Can you work these out from the model? Positions are in its coordinate system, mm. A direction names the side the tool comes from. Give positions to 0.01 mm unless a question says otherwise; leave off trailing zeros. Write each loop counter-clockwise with the first axis right and the second up, starting at its lowest first coordinate (ties: lowest second). Pieces come first, ordered by that corner, then holes.
from build123d import *

# Parameters (mm, degrees)
F0_W     = 50
F0_H     = 186
F1_DEPTH = 2
F2_W     = 50
F2_H     = 26
F2_R     = 5
F2_H_2   = 4
F3_DEPTH = 4
F4_W     = 50
F4_H     = 60
F5_DEPTH = 5


with BuildPart() as f1:
    # F0 (on Front) → F1 (new body, symmetric)
    with BuildSketch(Plane.XZ):
        with Locations((0.1773070544, -2)):
            Rectangle(F0_W, F0_H)
    extrude(amount=F1_DEPTH, both=True)

    # F2 (on face) → F3 (join)
    with BuildSketch(Plane.XY.offset(91)):
        with Locations((0.1773070544, 15)):
            Rectangle(F2_W, F2_H)
        with Locations((0.1773070544, 13)):
            Circle(F2_R, mode=Mode.SUBTRACT)
        with Locations((0.1773070544, 0)):
            Rectangle(F2_W, F2_H_2)
    extrude(amount=F3_DEPTH)

    # F4 (on face) → F5 (join)
    with BuildSketch(Plane.XZ.offset(2)):
        with Locations((0.1773070544, -65)):
            Rectangle(F4_W, F4_H)
    extrude(amount=F5_DEPTH)


solid = f1.part
(1) If I drill on L1, parallel to Z at x = -7.5, y = 24; L2, parallel to Y at x = 4.5, z = -31.5; L3, parallel to Y at x = -8, z = -75, over which ranges is the centre line in solid material (lowest first)?
Returned:
L1: z = 91 to 95
L2: y = -2 to 2
L3: y = -7 to 2
(2) Will these pins go through, and if not, where does the flat tip stop? P1, Ø6, axis at x = -5, z = -5.5, coming from the +Y side; P2, Ø10, axis at x = 11.5, z = 1, coming from the -Y side.
Returned:
P1: stops at y = 2
P2: stops at y = -2
(3) Imagine slicing it at B-B, the plane x = 1. Write out the boundary of the cut face in (y, z), plus the area to 3 significant figures.
Returned:
outline: (-7, -95) - (2, -95) - (2, 91) - (8.07, 91) - (8.07, 95) - (-2, 95) - (-2, -35) - (-7, -35) - close; (17.93, 91) - (28, 91) - (28, 95) - (17.93, 95) - close
area: 1,120 mm2
(4) For faces 1 (the face through (0, -2, 29)), 2 (the face through (-6, 15, 91)), 3 (the face through (0, -2, -95)), which set-ups out of +Z, -Z, +X, -X, +Y, -Y let a thin tool reach every point of the face, with its end or its side?
Returned:
face 1: +Z, +X, -X, -Y
face 2: -Z, +X, -X, +Y
face 3: -Z, +X, -X, +Y, -Y
(5) Imagine slicing it at A-A, the plane y = 13. Write out the boundary of the cut face in (x, z).
Returned:
outline: (-24.82, 91) - (-4.82, 91) - (-4.82, 95) - (-24.82, 95) - close; (5.18, 91) - (25.18, 91) - (25.18, 95) - (5.18, 95) - close
(6) Imagine slicing it at C-C, the plane x = 13.5. Write out the boundary of the cut face in (y, z), plus the area to 3 significant figures.
Returned:
outline: (-7, -95) - (2, -95) - (2, 91) - (28, 91) - (28, 95) - (-2, 95) - (-2, -35) - (-7, -35) - close
area: 1,160 mm2
(7) If we mould it in two halves opening along Y, with no side actions, what happens to faces 4 (the face through (0, -7, -65)), 5 (the face through (-0.474, 17.957, 92.972)), 6 (the face through (0, -4, -35)), 7 (the face through (0, 28, 93))? For each: +Y half, -Y half, draft (parallel to the pull), parting line (faces both ways), or undercut.
Returned:
face 4: -Y half
face 5: undercut
face 6: draft
face 7: +Y half
(8) Imagine slicing it at D-D, the plane z = -56. Write out the boundary of the cut face in (x, y), plus the area to 3 significant figures.
Returned:
outline: (-24.82, -7) - (25.18, -7) - (25.18, 2) - (-24.82, 2) - close
area: 450 mm2
